Source: CAD feature listing. Evaluate the final solid. Frame: model axes, mm. Face numbers are marked on the shaded views. A direction names the side the tool comes from. Round coordinates to 2 decimals unless told otherwise and drop trailing zeros. Order: outer loops, then holes, each group sorted by start corner. A loop starts at its lowest first (then second) coordinate and runs counter-clockwise, first axis right, second up. Notation, with made-up numbers: M 29,54.5 L 36,54.5 A30 ccw 36,77.5 Z; hole C -8,2.5 d1. An arc over 180 degrees is marked long. Answer as CSV lines item,"result". Start each with the question number.
Item 1: Line query: line 1 (Z direction, x = 0, y = -3.55); line 2 (X direction, y = 0, z = -10.75); line 3 (Z direction, x = 0, y = 5.5). Output: solid intervals per line, ascending. Write a range as [from, to].
Item 2: Section query C-C on z = -6. Return the cut outline in (x, y).
Item 3: Pull-direction query (Y, two-part tool) for the marked faces 1, 2 and 3; classes: +Y half, -Y half, draft (parallel to the pull), parting line (faces both ways), or undercut.
Item 4: Section query D-D on x = 1.5. Return the cut outline in (y, z).
Item 5: First-contact query: P1, Ø4, axis at y = 3, z = -12.5, coming from the +X side; P2, Ø1.5, axis at y = 1.5, z = -13.5, coming from the +X side. Flat tips, straight axial feed; report the tip coordinate or a pass-through.
Item 6: Set-up query: the marked faces 4 and 5. Return all of +Z, -Z, +X, -X, +Y, -Y with unobstructed straight access to the full face (end or side cutting, diameter ignored); none if empty.
Item 7: Section query A-A on x = 0. Return the cut outline in (y, z).
Item 8: Section query B-B on y = 0. Return the cut outline in (x, z).
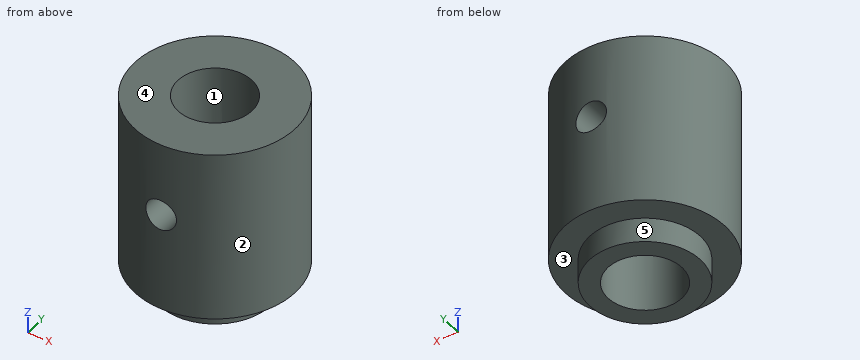
Autodesk Inventor part; units mm, degrees
ref_plane "Arbeitsebene1" through (0, 6.5, 0) normal (0, 1, 0) x (-1, 0, 0)
ref_plane "YZ Plane" through (0, 0, 0) normal (1, 0, 0) x (0, 1, 0)
ref_plane "XY Plane" through (0, 0, 0) normal (0, 0, 1) x (1, 0, 0)
sketch "Skizze1" plane through (0, 0, 0) normal (0, 1, 0) x (-1, 0, 0)
  line L0 (0, 0) -> (6.5, 0)
  line L1 (6.5, 0) -> (6.5, -14)
  line L2 (6.5, -14) -> (0, -14)
  line L3 (0, -14) -> (0, 0)
  point P0 (6.5, -7)
  dimension "d0" = 13
  dimension "d1" = 14
revolve "Umdrehung1" add sketch "Skizze1" angle 360 about axis through (0, 0, -14) along (0, 0, 1)
ref_plane "Arbeitsebene1" through (0, 6.5, 0) normal (0, 1, 0) x (-1, 0, 0)
sketch "Skizze3" plane through (0, 6.5, 0) normal (0, 1, 0) x (-1, 0, 0)
  point P0 (0, 0)
  point P1 (0, -6)
  dimension "d11" = 6
hole "Bohrung2" at (0, 6.5, -6) direction (0, -1, 0) diameter 2.5 end through all
sketch "Skizze6" plane through (0, 0, -14) normal (0, 0, -1) x (-1, 0, 0)
  circle A0 centre (0, 0) radius 4.5
  point P0 (0, 0)
extrude "Extrusion1" add sketch "Skizze6" along normal blind 2
sketch "Skizze4" plane through (0, 0, 0) normal (0, 0, 1) x (1, 0, 0)
  circle A0 centre (0, 0) radius 6.5
  point P0 (0, 0)
hole "Bohrung3" at (0, 0, 0) direction (0, 0, -1) diameter 6 end through all
properties part number "205 part 2" material "Gold"
Results:
1,line 1,"[-16, -7.25], [-4.75, 0]"
1,line 2,"[-6.5, -3], [3, 6.5]"
1,line 3,"[-14, -7.25], [-4.75, 0]"
2,outline,"M -1.25,-6.38 L -1.25,-2.73 A3 cw -1.25,2.73 L -1.25,6.38 A6.5 ccw Z; M 1.25,-6.38 A6.5 ccw 1.25,6.38 L 1.25,2.73 A3 cw 1.25,-2.73 Z"
3,face 1,"undercut"
3,face 2,"parting line"
3,face 3,"draft"
4,outline,"M -6.32,-14 L -4.24,-14 L -4.24,-16 L -2.6,-16 L -2.6,0 L -6.32,0 Z; M 2.6,-16 L 4.24,-16 L 4.24,-14 L 6.32,-14 L 6.32,0 L 2.6,0 Z"
5,P1,"x = 6.42"
5,P2,"x = 6.46"
6,face 4,"+Z, +X, -X, +Y, -Y"
6,face 5,"-Z"
7,outline,"M -6.5,-14 L -4.5,-14 L -4.5,-16 L -3,-16 L -3,-7.25 L -6.5,-7.25 Z; M -6.5,-4.75 L -3,-4.75 L -3,0 L -6.5,0 Z; M 3,-16 L 4.5,-16 L 4.5,-14 L 6.5,-14 L 6.5,-7.25 L 3,-7.25 Z; M 3,-4.75 L 6.5,-4.75 L 6.5,0 L 3,0 Z"
8,outline,"M -6.5,-14 L -4.5,-14 L -4.5,-16 L -3,-16 L -3,0 L -6.5,0 Z; M 3,-16 L 4.5,-16 L 4.5,-14 L 6.5,-14 L 6.5,0 L 3,0 Z"
